Job drawing, mm, ordinate dimensions from the low corner. One solid piece. A direction names the side the tool comes from. Give positions to 0.01 mm unless a question says otherwise; leave off trailing zeros. Loops run counter-clockwise (first coordinate to the right, second up) from the corner with the lowest first, then second, coordinate; pieces in that order, holes last. Notation, with made-up numbers: (35, -33) -> (93, -33) arc R9 cw to (93, -18) -> close; hole circle Ø3 at (85.5, -19.5). An arc over 180 degrees is marked (long way). Use one line per item in the form item = value.
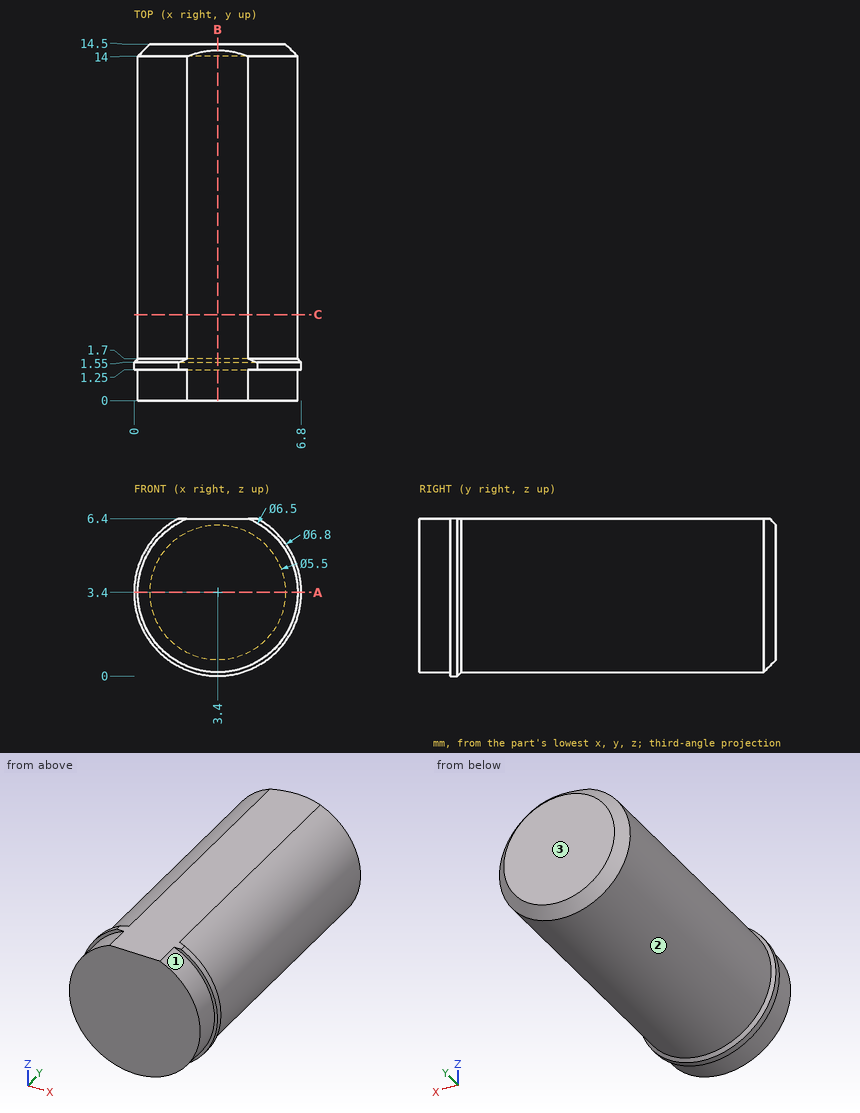
1. Drop flat-ended pins along their axis: P1, Ø2, axis at y = 3.5, z = 5.5, coming from the +X side; P2, Ø1.5, axis at y = 9.5, z = 4.5, coming from the -X side; P3, Ø1, axis at y = 10, z = 2.5, coming from the +X side. Give the stop position or say it passes through.
Result sheet:
P1 = 6.46
P2 = 0.17
P3 = 6.63
2. Cut at A-A, the plane z = 3.4. Write the cut outline in (x, y), then the cut area to 3 significant figures.
Result sheet:
outline = (0, 1.25) -> (0.15, 1.25) -> (0.15, 0) -> (6.65, 0) -> (6.65, 1.25) -> (6.8, 1.25) -> (6.8, 1.55) -> (6.65, 1.7) -> (6.65, 14) -> (6.15, 14.5) -> (0.65, 14.5) -> (0.15, 14) -> (0.15, 1.7) -> (0, 1.55) -> close
area = 94.1 mm^2
3. Drill centre lines: line 1 (X direction, y = 3.5, z = 3.5); line 2 (Z direction, x = 3.25, y = 3.75); line 3 (X direction, y = 1.75, z = 6). Where is each one in solid material? Low to high.
Result sheet:
line_1 = 0.15 to 6.65
line_2 = 0.15 to 6.4
line_3 = 1.45 to 5.35
4. Cut at B-B, the plane x = 3.4. Write the cut outline in (y, z), then the cut area to 3 significant figures.
Result sheet:
outline = (0, 0.15) -> (1.25, 0.15) -> (1.25, 0) -> (1.55, 0) -> (1.7, 0.15) -> (14, 0.15) -> (14.5, 0.65) -> (14.5, 6.15) -> (14.25, 6.4) -> (0, 6.4) -> close
area = 90.5 mm^2
5. Tool access for the marked faces 1, 2 and 3: list every direction of +Z, -Z, +X, -X, +Y, -Y with a clear straight run to the whole face (end or side of a thin tool).
Result sheet:
face_1 = -Y
face_2 = +Y
face_3 = +Z, -Z, +X, -X, +Y
6. Cut at C-C, the plane y = 3.5. Write the cut outline in (x, z).
Result sheet:
outline = (2.15, 6.4) arc R3.25 ccw (long way) to (4.65, 6.4) -> close
